```python
from build123d import *

# Parameters (mm, degrees)
ESBO_O1_R                = 8.3
RESSALTO_EXTRUS_O1_DEPTH = 1.5
RESSALTO_EXTRUS_O2_DEPTH = 6
ESBO_O3_W                = 2.8
ESBO_O3_H                = 2.8
CORTE_EXTRUS_O1_DEPTH    = 37.142080737
ESBO_O4_W                = 2.8
ESBO_O4_H                = 2.8
CORTE_EXTRUS_O2_DEPTH    = 53.08166664
ESBO_O6_W                = 5
ESBO_O6_H                = 25
RESSALTO_EXTRUS_O5_DEPTH = 7.5
ESBO_O7_W                = 2.8
ESBO_O7_H                = 2.8
CORTE_EXTRUS_O3_DEPTH    = 60
ESBO_O8_W                = 60
ESBO_O8_H                = 52.5
ESBO_O8_R                = 8.3
RESSALTO_EXTRUS_O6_DEPTH = 1.5
ESBO_O9_R                = 8.3
RESSALTO_EXTRUS_O7_DEPTH = 1.5


with BuildPart() as part:
    # Esboço1 → Ressalto-extrusão1 (new body)
    with BuildSketch(Plane.XY):
        Polygon((-25, -12.5), (-25, 12.5), (25, 12.5), (25, -12.5), (15, -12.5), (-15, -12.5), align=None)
        with Locations((-13, 0)):
            Circle(ESBO_O1_R, mode=Mode.SUBTRACT)
        with Locations(Location((13, 0, 0), (0, 0, 180))):
            Circle(ESBO_O1_R, mode=Mode.SUBTRACT)
    extrude(amount=RESSALTO_EXTRUS_O1_DEPTH)

    # Esboço2 → Ressalto-extrusão2 (add)
    with BuildSketch(Plane.XY.offset(1.5)):
        Polygon((-20, -12.5), (-25, -12.5), (-25, -2.5), (-22, -2.5), (-22, -9.5), (-15, -9.5), (-15, -12.5), align=None)
        Polygon((22, -2.5), (22, -9.5), (15, -9.5), (15, -12.5), (20, -12.5), (25, -12.5), (25, -2.5), align=None)
        Polygon((20, 12.5), (25, 12.5), (25, 2.5), (22, 2.5), (22, 9.5), (15, 9.5), (15, 12.5), align=None)
        Polygon((-22, 2.5), (-22, 9.5), (-15, 9.5), (-15, 12.5), (-20, 12.5), (-25, 12.5), (-25, 2.5), align=None)
    extrude(amount=RESSALTO_EXTRUS_O2_DEPTH)

    # Esboço3 → Corte-extrusão1 (cut, through all)
    with BuildSketch(Plane.XZ.offset(12.5)):
        with Locations((-20, 3.75)):
            Rectangle(ESBO_O3_W, ESBO_O3_H)
        with Locations((20, 3.75)):
            Rectangle(ESBO_O3_W, ESBO_O3_H)
    extrude(amount=-CORTE_EXTRUS_O1_DEPTH, mode=Mode.SUBTRACT)

    # Esboço4 → Corte-extrusão2 (cut, through all)
    with BuildSketch(Plane.ZY.offset(25)):
        with Locations((3.75, 7.5)):
            Rectangle(ESBO_O4_W, ESBO_O4_H)
        with Locations((3.75, -7.5)):
            Rectangle(ESBO_O4_W, ESBO_O4_H)
    extrude(amount=-CORTE_EXTRUS_O2_DEPTH, mode=Mode.SUBTRACT)

    # Esboço6 → Ressalto-extrusão5 (add)
    with BuildSketch(Plane(origin=(0, 0, 0), x_dir=(-1, 0, 0), z_dir=(0, 0, -1))):
        with Locations((-27.5, 0)):
            Rectangle(ESBO_O6_W, ESBO_O6_H)
        with Locations((27.5, 0)):
            Rectangle(ESBO_O6_W, ESBO_O6_H)
    extrude(amount=-RESSALTO_EXTRUS_O5_DEPTH)

    # Esboço7 → Corte-extrusão3 (cut)
    with BuildSketch(Plane(origin=(30, 0, 0), x_dir=(0, 0, -1), z_dir=(1, 0, 0))):
        with Locations((-3.75, -7.5)):
            Rectangle(ESBO_O7_W, ESBO_O7_H)
        with Locations((-3.75, 7.5)):
            Rectangle(ESBO_O7_W, ESBO_O7_H)
    extrude(amount=-CORTE_EXTRUS_O3_DEPTH, mode=Mode.SUBTRACT)

    # Esboço8 → Ressalto-extrusão6 (add)
    with BuildSketch(Plane(origin=(0, 0, 0), x_dir=(-1, 0, 0), z_dir=(0, 0, -1))):
        Rectangle(ESBO_O8_W, ESBO_O8_H)
        with Locations(Location((13, 0, 0), (0, 0, 180))):
            Circle(ESBO_O8_R, mode=Mode.SUBTRACT)
        with Locations((-13, 0)):
            Circle(ESBO_O8_R, mode=Mode.SUBTRACT)
    extrude(amount=-RESSALTO_EXTRUS_O6_DEPTH)

    # Esboço9 → Ressalto-extrusão7 (add, through all)
    with BuildSketch(Plane.XY.offset(1.5)):
        with Locations((-13, 0)):
            Circle(ESBO_O9_R)
        with Locations((13, 0)):
            Circle(ESBO_O9_R)
    extrude(amount=-RESSALTO_EXTRUS_O7_DEPTH)


solid = part.part
```
Part model, mm, in its own coordinate system. A direction names the side the tool comes from. Round coordinates to 2 decimals unless told otherwise and drop trailing zeros. Order: outer loops, then holes, each group sorted by start corner. A loop starts at its lowest first (then second) coordinate and runs counter-clockwise, first axis right, second up. Notation, with made-up numbers: M 88.25,69.25 L 136.25,69.25 A20 ccw 136.25,75.25 Z; hole C 75,-11 d8. An arc over 180 degrees is marked long. Put each result on its own line as item: value. Start each with the question number.
1. Drill centre lines: probe 1 along X at (y, z) = (2, 5.5); probe 2 along Y at (x, z) = (-17, 2); probe 3 along X at (y, z) = (-5, 6.75). Where is each one in solid material? Low to high. Write a range as [from, to].
2. Drop flat-ended pins along their axis: pin 1 (2 mm diameter, centred on y = -16.5, z = 3, fed in from +X); pin 2 (3.5 mm diameter, centred on x = -23, z = 5, fed in from +Y); pin 3 (1.4 mm diameter, centred on x = -24.5, z = 4.5, fed in from -Y); pin 4 (3 mm diameter, centred on x = 10, y = -4.5, fed in from -Z). Give the stop position or say it passes through.
3. Slice it at A-A on y = -7. List the corners of the cut face in (x, z), then the cut area to 3 significant figures.
4. Slice it at D-D on x = 2. List the corners of the cut face in (y, z), then the cut area to 4 significant figures.
5. Slice it at C-C on y = -16. List the corners of the cut face in (x, z).
6. Tool access for faces 4 (the face through (-22, 5, 4)), 5 (the face through (-26, 8.9, 4)), 6 (the face through (-20, 11, 5.15)): list every direction of +Z, -Z, +X, -X, +Y, -Y with a clear straight run to the whole face (end or side of a thin tool).
7. Two-plate mould, pull along X, no slides. Class faces 1 (the face through (-30, 0, 3)), 2 (the face through (-22, -12.5, 4)), 3 (the face through (20, 11, 2.35)): +X half, -X half, draft (parallel to the pull), parting line (faces both ways), or undercut.
8. Slice it at B-B on z = 6. List the corners of the cut face in (x, y).
Findings:
1. probe 1: [-30, -25], [25, 30]
1. probe 2: [-12.5, -9.5], [9.5, 12.5]
1. probe 3: [-30, -22], [22, 30]
2. pin 1: through
2. pin 2: y = 12.5
2. pin 3: y = -12.5
2. pin 4: z = 0
3. outline: M -30,0 L 30,0 L 30,2.35 L 22,2.35 L 22,1.5 L -22,1.5 L -22,2.35 L -30,2.35 Z; M -30,5.15 L -22,5.15 L -22,7.5 L -30,7.5 Z; M 22,5.15 L 30,5.15 L 30,7.5 L 22,7.5 Z
3. area: 141 mm2
4. outline: M -26.25,0 L 26.25,0 L 26.25,1.5 L -26.25,1.5 Z
4. area: 78.75 mm2
5. outline: M -30,0 L 30,0 L 30,1.5 L -30,1.5 Z
6. face 4: +Z
6. face 5: +X, -X
6. face 6: +Y, -Y
7. face 1: -X half
7. face 2: draft
7. face 3: undercut
8. outline: M -30,-12.5 L -15,-12.5 L -15,-9.5 L -22,-9.5 L -22,-2.5 L -25,-2.5 L -25,2.5 L -22,2.5 L -22,9.5 L -15,9.5 L -15,12.5 L -30,12.5 Z; M 15,-12.5 L 30,-12.5 L 30,12.5 L 15,12.5 L 15,9.5 L 22,9.5 L 22,2.5 L 25,2.5 L 25,-2.5 L 22,-2.5 L 22,-9.5 L 15,-9.5 Z
